from build123d import *

# Parameters (mm, degrees)
SKETCH1_W            = 270
SKETCH1_H            = 260
BOSS_EXTRUDE1_DEPTH  = 6
SKETCH2_R            = 2
SKETCH2_W            = 35
SKETCH2_H            = 60
CUT_EXTRUDE1_DEPTH   = 188.512666239
SKETCH3_R            = 17
CUT_EXTRUDE2_DEPTH   = 188.512666239
SKETCH4_R            = 2
CUT_EXTRUDE3_DEPTH   = 188.512666239
SKETCH5_R            = 2
CUT_EXTRUDE4_DEPTH   = 188.512666239
FILLET1_R            = 15
SKETCH6_R            = 12.5
CUT_EXTRUDE5_DEPTH   = 188.512666239
SKETCH8_R            = 1.75
CUT_EXTRUDE6_DEPTH   = 188.512666239
SKETCH9_R            = 12.5
CUT_EXTRUDE7_DEPTH   = 188.512666239
SKETCH10_W           = 103.406579867
SKETCH10_H           = 30
CUT_EXTRUDE8_DEPTH   = 188.512666239
FILLET2_R            = 10
FILLET2_OF_MIRROR3_R = 10
SKETCH11_R           = 1.6
SKETCH11_R_2         = 3.5
CUT_EXTRUDE9_DEPTH   = 188.512666239
SKETCH12_R           = 15
CUT_EXTRUDE10_DEPTH  = 188.512666239
FILLET3_R            = 5
FILLET4_R            = 5
SKETCH13_R           = 1.75
SKETCH13_R_2         = 2
CUT_EXTRUDE11_DEPTH  = 188.512666239


with BuildPart() as part:
    # Sketch1 → Boss-Extrude1 (new body)
    with BuildSketch(Plane.XY):
        Rectangle(SKETCH1_W, SKETCH1_H)
    extrude(amount=BOSS_EXTRUDE1_DEPTH)

    # Sketch2 → Cut-Extrude1 (cut, through all)
    with BuildSketch(Plane.XY.offset(6)):
        with Locations((-85, 15)):
            Circle(SKETCH2_R)
        with Locations((-61, 15)):
            Circle(SKETCH2_R)
        with Locations((-61, -15)):
            Circle(SKETCH2_R)
        with Locations((-85, -15)):
            Circle(SKETCH2_R)
        with Locations((-117.5, 0)):
            Rectangle(SKETCH2_W, SKETCH2_H)
    cut_extrude1 = extrude(amount=-CUT_EXTRUDE1_DEPTH, mode=Mode.SUBTRACT)

    # Sketch3 → Cut-Extrude2 (cut, through all)
    with BuildSketch(Plane.XY.offset(6)):
        with Locations((0, -103.5)):
            Circle(SKETCH3_R)
    cut_extrude2 = extrude(amount=-CUT_EXTRUDE2_DEPTH, mode=Mode.SUBTRACT)

    # Mirror1: Cut-Extrude1 across plane
    add(cut_extrude1.mirror(Plane(origin=(0, 0, 0), x_dir=(0, 0, 1), z_dir=(1, 0, 0))), mode=Mode.SUBTRACT)

    # Mirror2: Cut-Extrude2 across plane
    add(cut_extrude2.mirror(Plane.ZX), mode=Mode.SUBTRACT)

    # Sketch4 → Cut-Extrude3 (cut, through all)
    with BuildSketch(Plane.XY.offset(6)):
        with Locations((21.25, -103.5)):
            Circle(SKETCH4_R)
        with Locations((-21.25, -103.5)):
            Circle(SKETCH4_R)
    extrude(amount=-CUT_EXTRUDE3_DEPTH, mode=Mode.SUBTRACT)

    # Sketch5 → Cut-Extrude4 (cut, through all)
    with BuildSketch(Plane.XY.offset(6)):
        with Locations((79.206538854, -126.234773755)):
            Circle(SKETCH5_R)
        with Locations((79.206538854, -105.765226245)):
            Circle(SKETCH5_R)
        with Locations((101.138196901, -105.765226245)):
            Circle(SKETCH5_R)
        with Locations((101.138196901, -126.234773755)):
            Circle(SKETCH5_R)
    extrude(amount=-CUT_EXTRUDE4_DEPTH, mode=Mode.SUBTRACT)

    # Fillet1
    fillet1_edges = [part.edges().sort_by_distance(p)[0] for p in [
        (135, -130, 3),
        (-135, -130, 3),
        (-135, 130, 3),
        (135, 130, 3),
    ]]
    fillet(fillet1_edges, radius=FILLET1_R)

    # Sketch6 → Cut-Extrude5 (cut, through all)
    with BuildSketch(Plane.XY.offset(6)):
        with Locations((-115, 115)):
            Circle(SKETCH6_R)
    extrude(amount=-CUT_EXTRUDE5_DEPTH, mode=Mode.SUBTRACT)

    # Sketch8 → Cut-Extrude6 (cut, through all)
    with BuildSketch(Plane.XY.offset(6)):
        with Locations((49.5, 31.3)):
            Circle(SKETCH8_R)
        with Locations((9.5, 31.3)):
            Circle(SKETCH8_R)
        with Locations((9.5, 71.3)):
            Circle(SKETCH8_R)
        with Locations((49.5, 71.3)):
            Circle(SKETCH8_R)
        with Locations((-49.5, 31.3)):
            Circle(SKETCH8_R)
        with Locations((-9.5, 31.3)):
            Circle(SKETCH8_R)
        with Locations((-49.5, 71.3)):
            Circle(SKETCH8_R)
        with Locations((-9.5, 71.3)):
            Circle(SKETCH8_R)
    extrude(amount=-CUT_EXTRUDE6_DEPTH, mode=Mode.SUBTRACT)

    # Sketch9 → Cut-Extrude7 (cut, through all)
    with BuildSketch(Plane.XY.offset(6)):
        with Locations((115, 111.5)):
            Circle(SKETCH9_R)
    extrude(amount=-CUT_EXTRUDE7_DEPTH, mode=Mode.SUBTRACT)

    # Sketch10 → Cut-Extrude8 (cut, through all)
    with BuildSketch(Plane.XY.offset(6)):
        with Locations((83.296710066, 115)):
            Rectangle(SKETCH10_W, SKETCH10_H)
    cut_extrude8 = extrude(amount=-CUT_EXTRUDE8_DEPTH, mode=Mode.SUBTRACT)

    # Fillet2
    fillet2_edges = [part.edges().sort_by_distance(p)[0] for p in [
        (31.593420133, 100, 3),
        (31.593420133, 130, 3),
    ]]
    fillet(fillet2_edges, radius=FILLET2_R)

    # Mirror3: Cut-Extrude8 across plane
    add(cut_extrude8.mirror(Plane.ZY), mode=Mode.SUBTRACT)

    # Fillet2 of Mirror3
    fillet2_of_mirror3_edges = [part.edges().sort_by_distance(p)[0] for p in [
        (-31.593420133, 100, 3),
        (-31.593420133, 130, 3),
    ]]
    fillet(fillet2_of_mirror3_edges, radius=FILLET2_OF_MIRROR3_R)

    # Sketch11 → Cut-Extrude9 (cut, through all)
    with BuildSketch(Plane.XY.offset(6)):
        with Locations((-17.320508076, 113.5)):
            Circle(SKETCH11_R)
        with Locations((17.320508076, 113.5)):
            Circle(SKETCH11_R)
        with Locations((0, 83.5)):
            Circle(SKETCH11_R)
        with Locations((89, 90)):
            Circle(SKETCH11_R_2)
        with Locations((-89, 90)):
            Circle(SKETCH11_R_2)
        with Locations((121, -116)):
            Circle(SKETCH11_R_2)
        with Locations((-120, -115)):
            Circle(SKETCH11_R_2)
    extrude(amount=-CUT_EXTRUDE9_DEPTH, mode=Mode.SUBTRACT)

    # Sketch12 → Cut-Extrude10 (cut, through all)
    with BuildSketch(Plane.XY.offset(6)):
        with Locations((115, 111.5)):
            Circle(SKETCH12_R)
        with Locations((-115, 111.5)):
            Circle(SKETCH12_R)
    extrude(amount=-CUT_EXTRUDE10_DEPTH, mode=Mode.SUBTRACT)

    # Fillet3
    fillet3_edges = [part.edges().sort_by_distance(p)[0] for p in [
        (135, 100, 3),
        (-135, 100, 3),
    ]]
    fillet(fillet3_edges, radius=FILLET3_R)

    # Fillet4
    fillet4_edges = [part.edges().sort_by_distance(p)[0] for p in [
        (-100, 30, 3),
        (-100, -30, 3),
        (-135, -30, 3),
        (-135, 30, 3),
        (100, -30, 3),
        (100, 30, 3),
        (135, 30, 3),
        (135, -30, 3),
    ]]
    fillet(fillet4_edges, radius=FILLET4_R)

    # Sketch13 → Cut-Extrude11 (cut, through all)
    with BuildSketch(Plane.XY.offset(6)):
        with Locations((33.544641935, -34.940258228)):
            Circle(SKETCH13_R)
        with Locations((73.544641935, -34.940258228)):
            Circle(SKETCH13_R)
        with Locations((73.544641935, -74.940258228)):
            Circle(SKETCH13_R)
        with Locations((33.544641935, -74.940258228)):
            Circle(SKETCH13_R)
        with Locations(Location((-33.544641935, -74.940258228, 0), (0, 0, 180))):
            Circle(SKETCH13_R)
        with Locations(Location((-73.544641935, -74.940258228, 0), (0, 0, 180))):
            Circle(SKETCH13_R)
        with Locations(Location((-73.544641935, -34.940258228, 0), (0, 0, 180))):
            Circle(SKETCH13_R)
        with Locations(Location((-33.544641935, -34.940258228, 0), (0, 0, 180))):
            Circle(SKETCH13_R)
        with Locations((-131, -100)):
            Circle(SKETCH13_R_2)
        with Locations((-131, -65)):
            Circle(SKETCH13_R_2)
        with Locations((-131, -30)):
            Circle(SKETCH13_R_2)
        with Locations((-131, 5)):
            Circle(SKETCH13_R_2)
        with Locations((-131, 40)):
            Circle(SKETCH13_R_2)
        with Locations((-131, 75)):
            Circle(SKETCH13_R_2)
        with Locations((-105, -126)):
            Circle(SKETCH13_R_2)
        with Locations((-55, -126)):
            Circle(SKETCH13_R_2)
        with Locations((-5, -126)):
            Circle(SKETCH13_R_2)
        with Locations((45, -126)):
            Circle(SKETCH13_R_2)
        with Locations((95, -126)):
            Circle(SKETCH13_R_2)
        with Locations((145, -126)):
            Circle(SKETCH13_R_2)
        with Locations((195, -126)):
            Circle(SKETCH13_R_2)
        with Locations((245, -126)):
            Circle(SKETCH13_R_2)
        with Locations((295, -126)):
            Circle(SKETCH13_R_2)
        with Locations((345, -126)):
            Circle(SKETCH13_R_2)
        with Locations((395, -126)):
            Circle(SKETCH13_R_2)
        with Locations((445, -126)):
            Circle(SKETCH13_R_2)
        with Locations((495, -126)):
            Circle(SKETCH13_R_2)
        with Locations(Location((131, 75, 0), (0, 0, 180))):
            Circle(SKETCH13_R_2)
        with Locations(Location((131, 40, 0), (0, 0, 180))):
            Circle(SKETCH13_R_2)
        with Locations((131, 5)):
            Circle(SKETCH13_R_2)
        with Locations((131, -30)):
            Circle(SKETCH13_R_2)
        with Locations(Location((131, -65, 0), (0, 0, 180))):
            Circle(SKETCH13_R_2)
        with Locations(Location((131, -100, 0), (0, 0, 180))):
            Circle(SKETCH13_R_2)
    extrude(amount=-CUT_EXTRUDE11_DEPTH, mode=Mode.SUBTRACT)


solid = part.part
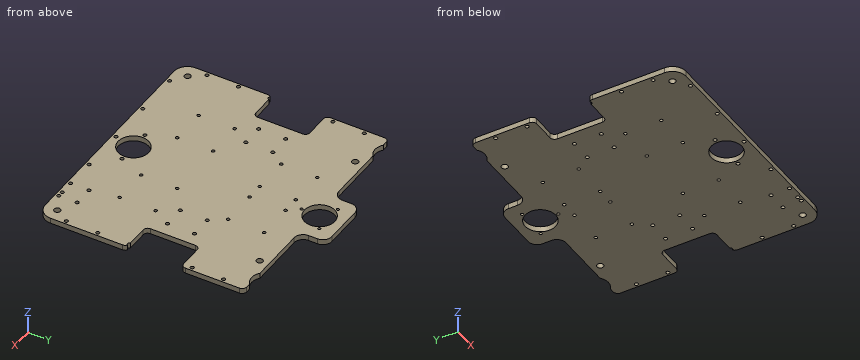
Geometry: final body of the model. Coordinates: model frame, mm. Round coordinates to 2 decimals unless told otherwise and drop trailing zeros. Order: outer loops, then holes, each group sorted by start corner. A loop starts at its lowest first (then second) coordinate and runs counter-clockwise, first axis right, second up. Notation, with made-up numbers: (5, -28.5) - (34, -28.5) arc R23 ccw to (34, 10.5) - close; hole circle Ø6 at (-34, 44). An arc over 180 degrees is marked (long way). Write each question's results on one line, items separated by ' | '.
Item 1: Section A-A, the plane y = -0.5. Return the cut outline in (x, z), and give its area (3 significant figures).
Completed:
outline: (-100, 0) - (100, 0) - (100, 6) - (-100, 6) - close | area: 1,200 mm^2
Item 2: First-contact query: pin 1 Ø4 at (x, y) = (89, 90) entering from +Z; pin 2 Ø2.5 at (x, z) = (-128, 2.5) entering from +Y. Flat tips, straight axial feed; report the tip coordinate or a pass-through.
Completed:
pin 1: through | pin 2: y = 100
Item 3: Section B-B, the plane z = 1.85. State how many separate pieces and enclosed holes the cut face has, and give its area (3 significant figures).
Completed:
separate pieces: 1 | enclosed holes: 52 | area: 57,100 mm^2
Item 4: Material intervals for line 1 along Y through (x, z) = (79, 4.25); line 2 along Y through (x, z) = (61, 4.15); line 3 along Y through (x, z) = (115.5, 5), sorted ascending. Write a range as [from, to].
Completed:
line 1: [-130, -128.22], [-124.25, -107.75], [-103.78, 100] | line 2: [-130, -17], [-13, 13], [17, 100] | line 3: [-130, -30], [30, 96.51]
